from build123d import *

# Parameters (mm, degrees)
F0_W     = 203.2
F0_H     = 3.175
F2_W     = 6.35
F2_H     = 6.35
F3_DEPTH = 12.7
F4_W     = 1.5875
F4_H     = 6.35
F5_DEPTH = 19.05
F6_R     = 1.5875
F7_DEPTH = 25.4


with BuildPart() as f1:
    # F0 (on Front) → F1 (revolve)
    with BuildSketch(Plane.XZ):
        with Locations((0, 1.5875)):
            Rectangle(F0_W, F0_H)
    revolve(axis=Axis((0, 0, 0), (1, 0, 0)))

    # F2 (on face) → F3 (join)
    with BuildSketch(Plane(origin=(-101.6, 0, 0), x_dir=(0, -1, 0), z_dir=(-1, 0, 0))):
        Rectangle(F2_W, F2_H)
    extrude(amount=F3_DEPTH)

    # F4 (on face) → F5 (join)
    with BuildSketch(Plane(origin=(-114.3, 0, 0), x_dir=(0, -1, 0), z_dir=(-1, 0, 0))):
        with Locations((2.38125, 0)):
            Rectangle(F4_W, F4_H)
        with Locations((-2.38125, 0)):
            Rectangle(F4_W, F4_H)
    extrude(amount=F5_DEPTH)

    # F6 (on face) → F7 (cut)
    with BuildSketch(Plane.XZ.offset(3.175)):
        with Locations((-129.2225, 0)):
            Circle(F6_R)
    extrude(amount=-F7_DEPTH, mode=Mode.SUBTRACT)


solid = f1.part
Here's how the part is built. I have some questions about the finished solid (model axes, mm). A direction names the side the tool comes from. Round coordinates to 2 decimals unless told otherwise and drop trailing zeros. Loops run counter-clockwise (first coordinate to the right, second up) from the corner with the lowest first, then second, coordinate; pieces in that order, holes last. Notation, with made-up numbers: (46.5, -21.75) - (77.5, -21.75) arc R21 ccw to (77.5, 14.25) - close; hole circle Ø2 at (82.25, 7). An arc over 180 degrees is marked (long way). One line per question, with ' | ' between items. Start each with the question number.
Q1. Please list where these lines run through material, in increasing order: line 1 (Y direction, x = -64.5, z = 2.75); line 2 (Y direction, x = -64.5, z = 0.5); line 3 (X direction, y = 0.5, z = 1.25). Write a range as [from, to].
Q2. Will this pin go through, and if not, where does the flat tip stop? pin 1 (1 mm diameter, centred on y = 0.5, z = -1, fed in from -X).
Q3. For faces 4 (the flat face through (101.6, 0, 0)), 5 (the cylindrical face through (1.42, 3.1, -0.69)), 6 (the flat face through (-124, -1.588, 0)), which set-ups out of +Z, -Z, +X, -X, +Y, -Y let a thin tool reach every point of the face, with its end or its side?
Q4. I want a section at A-A (x = 58). Write out the boundary of the cut face in (y, z) (3 decimals), then the cut area to 3 significant figures.
Q5. We'd pull the mould along Y, two halves only. Please class faces 1 (the flat face through (-117, 3.175, 0)), 2 (the flat face through (-117, -3.175, 0)), 3 (the flat face through (-124, 1.588, 0)): +Y half, -Y half, draft (parallel to the pull), parting line (faces both ways), or undercut.
Response values:
1) line 1: y = [-1.59, 1.59] | line 2: y = [-3.14, 3.14] | line 3: x = [-114.3, 101.6]
2) pin 1: stops at x = -114.3
3) face 4: +Z, -Z, +X, +Y, -Y | face 5: +X | face 6: +Z, -Z, -X
4) outline: circle Ø6.35 at (0, 0) | area: 31.7 mm²
5) face 1: +Y half | face 2: -Y half | face 3: undercut
